Answer from the drawing. Dimensions are ordinates in mm from the lowest x, y and z of the part. Coordinates: 2 decimals unless noted, no trailing zeros. Write each loop counter-clockwise with the first axis right and the second up, starting at its lowest first coordinate (ties: lowest second). Pieces come first, ordered by that corner, then holes. Notation, with made-up numbers: (-20, 31) -> (39, 31) arc R8 cw to (39, 39) -> close; hole circle Ø9 at (20.5, 71). An arc over 180 degrees is marked (long way). Answer as a JSON object with one key per item and string values. Group by question number.
(1) Straight lines are drawn through the part: L1, parallel to Z at x = 343, y = 11.25; L2, parallel to Z at x = 38.5, y = 4.5. For each, find the intervals that lie inside material, in ascending order.
(2) Flat-ended cylindrical pins translate along their axes: P1, Ø10, axis at y = 5.5, z = 284, coming from the -X side; P2, Ø2, axis at x = 344.5, y = 3.5, coming from the -Z side. Find the tip coordinate at first contact, or state that the pin passes through.
(3) Find section A-A (y = 12). Give the vertices of the cut face in (x, z).
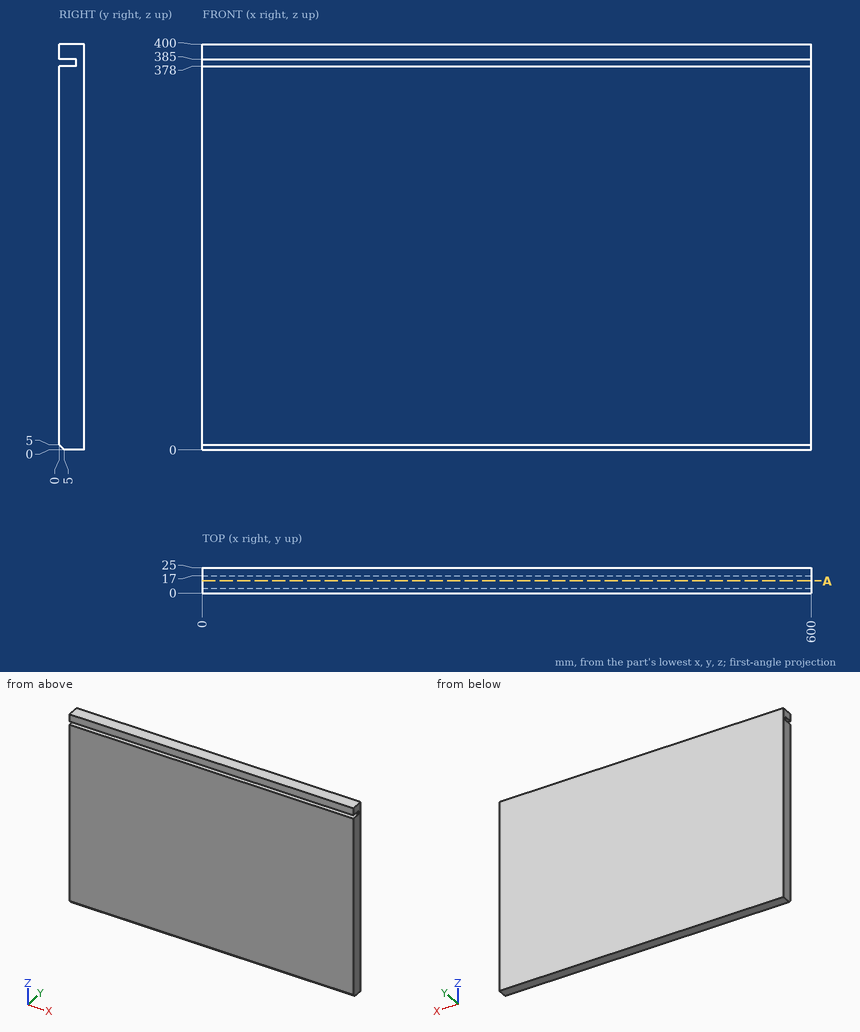
Results below:
{
 "1": {"L1": "z = 0 to 378, 385 to 400", "L2": "z = 0.5 to 378, 385 to 400"},
 "2": {"P1": "stops at x = 0", "P2": "stops at z = 0.5"},
 "3": {"outline": "(0, 0) -> (600, 0) -> (600, 378) -> (0, 378) -> close; (0, 385) -> (600, 385) -> (600, 400) -> (0, 400) -> close"}
}
